For this review, take the finished solid that the model builds, in its own axes (mm). Face numbers are marked on the shaded views. A direction names the side the tool comes from. Give positions to 0.01 mm unless a question says otherwise; leave off trailing zeros. Write each loop counter-clockwise with the first axis right and the second up, starting at its lowest first coordinate (ties: lowest second). Pieces come first, ordered by that corner, then holes. Notation, with made-up numbers: M -17,15.5 L -3,15.5 A28 cw -3,33.5 Z; hole C 21,21.25 d7. An arc over 180 degrees is marked long. One line per item, written item: value. Start each with the question number.
Item 1: Consider section B-B, the plane z = 10. Write out the cut boundary in (x, y).
Item 2: Consider section C-C, the plane x = 5.5. Write out the cut boundary in (y, z), and give its area (3 significant figures).
Item 3: Clearance check with flat-ended pins moving along their axes: pin 1 Ø4 at (x, z) = (2, 7) entering from -Y; pin 2 Ø5 at (y, z) = (16, 10) entering from -X; pin 3 Ø2 at (x, z) = (3.5, 15) entering from +Y. State where each tip first meets the part, or that it passes through.
Item 4: Mouldability with a two-part tool opening along Z and no side actions: class the marked faces 1, 2 and 3 as released by +Z, released by -Z, zero draft, split by the parting line, or undercut.
Item 5: Consider section D-D, the plane z = 4.75. Write out the cut boundary in (x, y).
Item 6: Consider section A-A, the plane y = 16. Write out the cut boundary in (x, z).
Item 7: Tool access review of the marked faces 4 and 5: name each direction out of +Z, -Z, +X, -X, +Y, -Y from which nothing blocks a thin tool from reaching the whole face with its end or side.
Item 8: To check wall thickness, follow probe 1 along X at (y, z) = (18.5, 2.25); probe 2 along Z at (x, y) = (-6.3, 16); probe 3 along Y at (x, z) = (-7.55, 10). State the ranges of each line that lie inside material, in increasing order.
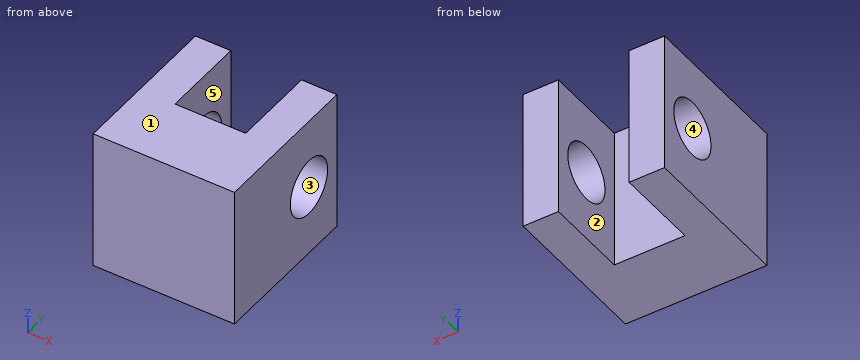
```python
from build123d import *

# Parameters (mm, degrees)
BOSS_EXTRU_1_DEPTH           = 20
ENL_V_MAT_EXTRU_1_DEPTH      = 34.301651611
ENL_V_MAT_EXTRU_1_DEPTH_BACK = 34.301651611
ESQUISSE2_R                  = 4


with BuildPart() as part:
    # Esquisse1 → Boss.-Extru.1 (new body)
    with BuildSketch(Plane.XY):
        Polygon((-10, 0), (10, 0), (10, 22), (5, 22), (5, 10), (-5, 10), (-5, 22), (-10, 22), align=None)
    extrude(amount=BOSS_EXTRU_1_DEPTH)

    # Esquisse2 → Enlèv. mat.-Extru.1 (cut, two sides: drawn at the far end of the back side and taken through both)
    with BuildSketch(Plane(origin=(-5, 0, 0), x_dir=(0, 0, -1), z_dir=(1, 0, 0)).offset(-ENL_V_MAT_EXTRU_1_DEPTH_BACK)):
        with Locations(Location((-10, 16, 0), (0, 0, 90))):
            Circle(ESQUISSE2_R)
    extrude(amount=ENL_V_MAT_EXTRU_1_DEPTH + ENL_V_MAT_EXTRU_1_DEPTH_BACK, mode=Mode.SUBTRACT)


solid = part.part
```
Model answer:
1. outline: M -10,0 L 10,0 L 10,12 L 5,12 L 5,10 L -5,10 L -5,12 L -10,12 Z; M -10,20 L -5,20 L -5,22 L -10,22 Z; M 5,20 L 10,20 L 10,22 L 5,22 Z
2. outline: M 0,0 L 22,0 L 22,20 L 0,20 Z; hole C 16,10 d8
2. area: 390 mm2
3. pin 1: stops at y = 0
3. pin 2: passes through
3. pin 3: stops at y = 10
4. face 1: released by +Z
4. face 2: zero draft
4. face 3: undercut
5. outline: M -10,0 L 10,0 L 10,22 L 5,22 L 5,10 L -5,10 L -5,22 L -10,22 Z
6. outline: M -10,0 L -5,0 L -5,6 L -10,6 Z; M -10,14 L -5,14 L -5,20 L -10,20 Z; M 5,0 L 10,0 L 10,6 L 5,6 Z; M 5,14 L 10,14 L 10,20 L 5,20 Z
7. face 4: +X, -X
7. face 5: +Z, -Z, +Y
8. probe 1: x = -10 to -5, 5 to 10
8. probe 2: z = 0 to 6, 14 to 20
8. probe 3: y = 0 to 12, 20 to 22
